The model under review builds one solid part; all positions refer to its coordinate system, in mm. Face numbers are marked on the shaded views. A direction names the side the tool comes from. Coordinates: 2 decimals unless noted, no trailing zeros. Write each loop counter-clockwise with the first axis right and the second up, starting at its lowest first coordinate (ties: lowest second). Pieces come first, ordered by that corner, then holes. Notation, with made-up numbers: M 72,14.5 L 111,14.5 A28 ccw 111,38.5 Z; hole C -4,31 d1. An arc over 180 degrees is marked long. Answer as a JSON object with one key per item and string values.
```python
from build123d import *

# Parameters (mm, degrees)
SKETCH003_W  = 16
SKETCH003_H  = 15
PAD_DEPTH    = 2.5
SKETCH_W     = 40
SKETCH_H     = 15
SKETCH_R     = 3.1
PAD001_DEPTH = 3
FILLET_R     = 1.5


with BuildPart() as part:
    # Sketch003 → Pad (new body)
    with BuildSketch(Plane.XY.offset(12)):
        with Locations((8, -7.5)):
            Rectangle(SKETCH003_W, SKETCH003_H)
    extrude(amount=PAD_DEPTH)

    # Sketch → Pad001 (new body)
    with BuildSketch(Plane.XY.offset(14.5)):
        with Locations((8, -7.5)):
            Rectangle(SKETCH_W, SKETCH_H)
        with Locations((-6, -7.5)):
            Circle(SKETCH_R, mode=Mode.SUBTRACT)
        with Locations((22, -7.5)):
            Circle(SKETCH_R, mode=Mode.SUBTRACT)
    extrude(amount=PAD001_DEPTH)

    # Fillet
    fillet_edges = [part.edges().sort_by_distance(p)[0] for p in [
        (8, 0, 17.5),
        (8, -15, 17.5),
        (-12, -7.5, 17.5),
        (28, -7.5, 17.5),
    ]]
    fillet(fillet_edges, radius=FILLET_R)


solid = part.part
```
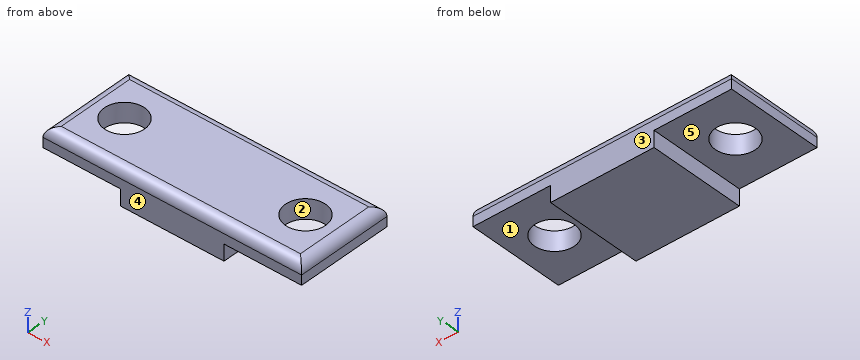
(1) Add section A-A on x = 22. Give the boundary of the cut face in (y, z), and give its area (3 significant figures).
Results list:
{"outline": "M -15,14.5 L -10.6,14.5 L -10.6,17.5 L -13.5,17.5 A1.5 ccw -15,16 Z; M -4.4,14.5 L 0,14.5 L 0,16 A1.5 ccw -1.5,17.5 L -4.4,17.5 Z", "area": "25.4 mm²"}
(2) Draft analysis for pull direction Y (two halves, no side actions). For the marked faces 1, 2 and 3, state which applies: released by +Y, released by -Y, zero draft, split by the parting line, or undercut.
Results list:
{"face 1": "zero draft", "face 2": "undercut", "face 3": "released by +Y"}
(3) Wall thickness on line 1 along Y through (x, z) = (-6, 15.6); line 2 along Z through (x, y) = (24, -11); line 3 along X through (y, z) = (-10.75, 14.1): over which ranges is each line inside the solid? List them lowest first. Write a range as from..to.
Results list:
{"line 1": "-15..-10.6, -4.4..0", "line 2": "14.5..17.5", "line 3": "0..16"}
(4) Add section B-B on y = -7.5. Give the boundary of the cut face in (x, z), and give its area (3 significant figures).
Results list:
{"outline": "M -12,14.5 L -9.1,14.5 L -9.1,17.5 L -10.5,17.5 A1.5 ccw -12,16 Z; M -2.9,14.5 L 0,14.5 L 0,12 L 16,12 L 16,14.5 L 18.9,14.5 L 18.9,17.5 L -2.9,17.5 Z; M 25.1,14.5 L 28,14.5 L 28,16 A1.5 ccw 26.5,17.5 L 25.1,17.5 Z", "area": "122 mm²"}
(5) For pin 1 Ø7 at (x, y) = (22, -7.5) entering from -Z; pin 2 Ø2 at (y, z) = (-9.5, 13) entering from -X, all flat-tipped, find the tip position at first contact; note any pin that passes through.
Results list:
{"pin 1": "z = 14.5", "pin 2": "x = 0"}
(6) Add section C-C on z = 15.55. Give the boundary of the cut face in (x, y), and give its area (3 significant figures).
Results list:
{"outline": "M -12,-15 L 28,-15 L 28,0 L -12,0 Z; hole C -6,-7.5 d6.2; hole C 22,-7.5 d6.2", "area": "540 mm²"}
(7) For the marked faces 4 and 5, list the 3-axis set-ups (+Z, -Z, +X, -X, +Y, -Y) from which the entire face can be reached by the end or side of a thin tool; tool diameter is ignored.
Results list:
{"face 4": "+Z, -Z, +X, -X, -Y", "face 5": "-Z, -X, +Y, -Y"}
(8) Add section D-D on x = -7. Give the boundary of the cut face in (y, z), and give its area (3 significant figures).
Results list:
{"outline": "M -15,14.5 L -10.43,14.5 L -10.43,17.5 L -13.5,17.5 A1.5 ccw -15,16 Z; M -4.57,14.5 L 0,14.5 L 0,16 A1.5 ccw -1.5,17.5 L -4.57,17.5 Z", "area": "26.4 mm²"}
